Check sheet for the modelled part. Datum: model origin and axes. Units: mm. Give positions to 0.01 mm unless a question says otherwise; leave off trailing zeros. Order: outer loops, then holes, each group sorted by start corner. A loop starts at its lowest first (then second) coordinate and runs counter-clockwise, first axis right, second up.
```python
from build123d import *

# Parameters (mm, degrees)
SKETCH1_W           = 380
SKETCH1_H           = 294.5
SKETCH1_R           = 11
SKETCH1_R_2         = 1.5
BOSS_EXTRUDE1_DEPTH = 3
FILLET1_R           = 3


with BuildPart() as part:
    # Sketch1 → Boss-Extrude1 (new body)
    with BuildSketch(Plane.XY):
        Rectangle(SKETCH1_W, SKETCH1_H)
        with Locations((-172.5, 129.75)):
            Circle(SKETCH1_R, mode=Mode.SUBTRACT)
        with Locations(Location((172.5, 129.75, 0), (0, 0, 180))):
            Circle(SKETCH1_R, mode=Mode.SUBTRACT)
        with Locations((172.5, -129.75)):
            Circle(SKETCH1_R, mode=Mode.SUBTRACT)
        with Locations(Location((-172.5, -129.75, 0), (0, 0, 180))):
            Circle(SKETCH1_R, mode=Mode.SUBTRACT)
        with Locations((150.5, 138.25)):
            Circle(SKETCH1_R_2, mode=Mode.SUBTRACT)
        with Locations((-186.5, 102.25)):
            Circle(SKETCH1_R_2, mode=Mode.SUBTRACT)
        with Locations((-150.5, -138.25)):
            Circle(SKETCH1_R_2, mode=Mode.SUBTRACT)
        with Locations((186.5, -102.25)):
            Circle(SKETCH1_R_2, mode=Mode.SUBTRACT)
    extrude(amount=BOSS_EXTRUDE1_DEPTH)

    # Fillet1
    fillet1_edges = [part.edges().sort_by_distance(p)[0] for p in [
        (-190, 147.25, 1.5),
        (190, 147.25, 1.5),
        (190, -147.25, 1.5),
        (-190, -147.25, 1.5),
    ]]
    fillet(fillet1_edges, radius=FILLET1_R)


solid = part.part
```
(1) Cross-section at B-B on x = 172.5. Enter the section's corners in (y, z).
Response values:
outline: (-147.25, 0) - (-140.75, 0) - (-140.75, 3) - (-147.25, 3) - close; (-118.75, 0) - (118.75, 0) - (118.75, 3) - (-118.75, 3) - close; (140.75, 0) - (147.25, 0) - (147.25, 3) - (140.75, 3) - close
(2) Release check for a two-part mould opening along Y. For faces 1 (the face through (-3, 2, 3)), 2 (the face through (161.51, -129.27, 1.48)), 3 (the face through (183.49, 129.27, 1.48)) record: released by +Y, released by -Y, zero draft, split by the parting line, or undercut.
Response values:
face 1: zero draft
face 2: undercut
face 3: undercut
(3) Cross-section at A-A on y = -129.75. Enter the section's corners in (x, z).
Response values:
outline: (-190, 0) - (-183.5, 0) - (-183.5, 3) - (-190, 3) - close; (-161.5, 0) - (161.5, 0) - (161.5, 3) - (-161.5, 3) - close; (183.5, 0) - (190, 0) - (190, 3) - (183.5, 3) - close
(4) Material ranges on L1, parallel to Y at x = 172.5, z = 1.9; L2, parallel to Y at x = 164.5, z = 1.6; L3, parallel to Y at x = -186.5, z = 1.8, recorded low to high.
Response values:
L1: y = -147.25 to -140.75, -118.75 to 118.75, 140.75 to 147.25
L2: y = -147.25 to -137.3, -122.2 to 122.2, 137.3 to 147.25
L3: y = -147.25 to 100.75, 103.75 to 147.25
(5) Gauge pin test, flat end, axial feed: pin 1 Ø20 at (x, y) = (172.5, -129.75) entering from -Z. Record the tip position at first contact, or that the pin passes through.
Response values:
pin 1: passes through
